Part model, mm, in its own coordinate system. Face numbers are marked on the shaded views. A direction names the side the tool comes from. Coordinates: 2 decimals unless noted, no trailing zeros. Order: outer loops, then holes, each group sorted by start corner. A loop starts at its lowest first (then second) coordinate and runs counter-clockwise, first axis right, second up. Notation, with made-up numbers: M 72,70 L 102,70 A5 ccw 102,76 Z; hole C 31.5,21 d3. An arc over 180 degrees is marked long. Write item = value, one per line. Start each with the question number.
Autodesk Inventor part; units mm, degrees
ref_plane "YZ Plane" through (0, 0, 0) normal (1, 0, 0) x (0, 1, 0)
ref_plane "XZ Plane" through (0, 0, 0) normal (0, 1, 0) x (-1, 0, 0)
ref_plane "XY Plane" through (0, 0, 0) normal (0, 0, 1) x (1, 0, 0)
sketch "Skizze1" plane through (0, 0, 0) normal (0, 1, 0) x (-1, 0, 0)
  line L0 (-10, -5.25) -> (10, -5.25)
  line L1 (10, -5.25) -> (10, 5.25)
  line L2 (10, 5.25) -> (-10, 5.25)
  line L3 (-10, 5.25) -> (-10, -5.25)
  line L4 (-10, -5.25) -> (10, 5.25) construction
  line L5 (10, -5.25) -> (-10, 5.25) construction
  circle A0 centre (4.75, 2.25) radius 1.25
  circle A1 centre (-4.75, 2.25) radius 1.25
  point P0 (0, 0)
  dimension "d0" = 20
  dimension "d1" = 10.5
  dimension "d4" = 2.5
  dimension "d5" = 2.5
  dimension "d6" = 4.75
  dimension "d7" = 3
  dimension "d8" = 3
  dimension "d9" = 4.75
extrude "Extrusion1" add sketch "Skizze1" along normal mid plane 6
sketch "Skizze2" plane through (0, 0, 0) normal (0, 1, 0) x (-1, 0, 0)
  line L0 (10, -5.25) -> (10, 5.25)
  line L1 (10, 5.25) -> (-10, 5.25)
  line L2 (-10, 5.25) -> (-10, -5.25)
  line L3 (-10, -5.25) -> (10, -5.25)
  circle A0 centre (4.75, 2.25) radius 1.25
  circle A1 centre (-4.75, 2.25) radius 1.25
  line L4 (10, 5.25) -> (-10, 5.25)
  line L5 (8.2, 5.25) -> (7.7, 5.25)
  line L6 (7.7, 5.25) -> (7.7, 9.25)
  line L7 (7.7, 9.25) -> (8.2, 9.25)
  line L8 (8.2, 9.25) -> (8.2, 5.25)
  line L9 (0.3746, 5.25) -> (-0.1254, 5.25)
  line L10 (-0.1254, 5.25) -> (-0.1254, 9.25)
  line L11 (-0.1254, 9.25) -> (0.3746, 9.25)
  line L12 (0.3746, 9.25) -> (0.3746, 5.25)
  line L13 (-7.7, 5.25) -> (-8.2, 5.25)
  line L14 (-8.2, 5.25) -> (-8.2, 9.25)
  line L15 (-8.2, 9.25) -> (-7.7, 9.25)
  line L16 (-7.7, 9.25) -> (-7.7, 5.25)
  point P0 (0, 0)
  dimension "d10" = 0.5
  dimension "d11" = 4
  dimension "d12" = 1.8
  dimension "d13" = 1.8
  dimension "d14" = 0.5
  dimension "d15" = 0.5
extrude "Extrusion2" add sketch "Skizze2" along normal mid plane 3.2 contours L1 L6 L7 L8 | L14 L15 L16 L1 | L1 L10 L11 L12
sketch "Skizze3" plane through (0, 0, 0) normal (0, 1, 0) x (-1, 0, 0)
  line L0 (10, -5.25) -> (10, 5.25)
  line L1 (10, 5.25) -> (-10, 5.25)
  line L2 (-10, 5.25) -> (-10, -5.25)
  line L3 (-10, -5.25) -> (10, -5.25)
  circle A0 centre (4.75, 2.25) radius 1.25
  circle A1 centre (-4.75, 2.25) radius 1.25
  line L4 (10, -5.25) -> (-10, -5.25)
  line L5 (-7.1, -5.25) -> (9.9766, -10.265)
  line L6 (9.9766, -10.265) -> (9.1627, -13.0362)
  line L7 (9.1627, -13.0362) -> (10.7453, -13.501)
  line L8 (10.7453, -13.501) -> (11.7, -10.25)
  line L9 (11.7, -10.25) -> (-5.3255, -5.25)
  point P0 (0, 0)
  dimension "d18" = 2.9
  dimension "d19" = 0.5
  dimension "d20" = 1.7
  dimension "d21" = 5
extrude "Extrusion3" add sketch "Skizze3" along normal mid plane 3.4 contours L9 L8 L7 L6 L5 L3
sketch "Skizze4" plane through (0, 0, 0) normal (0, 1, 0) x (-1, 0, 0)
  line L0 (11.7, -10.25) -> (-5.3255, -5.25)
  line L1 (-7.1, -5.25) -> (-5.3255, -5.25)
  line L2 (-7.1, -5.25) -> (9.9766, -10.265)
  line L3 (9.9766, -10.265) -> (9.1627, -13.0362)
  line L4 (9.1627, -13.0362) -> (10.7453, -13.501)
  line L5 (10.7453, -13.501) -> (11.7, -10.25)
  circle A0 centre (10.3631, -11.8755) radius 2.3
  point P0 (0, 0)
  dimension "d24" = 4.6
extrude "Extrusion4" add sketch "Skizze4" along normal mid plane 3 contours L5 L4 L3 L2 A0 L0 | L0 A0 L2 L3 L4 L5
properties part number "00_Endstop_mechanical_vuniversum_microswitch_roll"
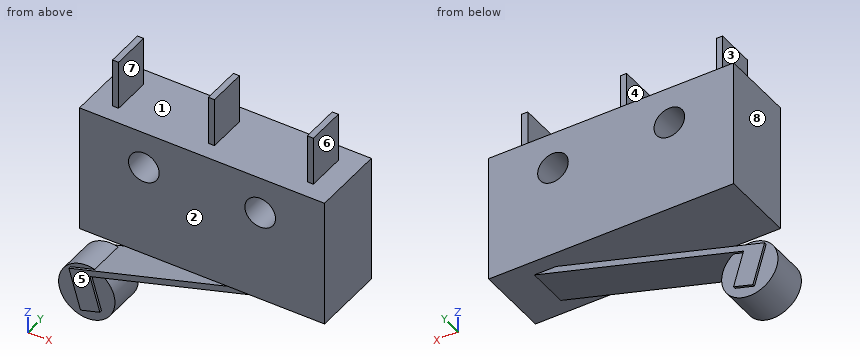
Item 1: Cut at C-C, the plane y = -2.3. Write the cut outline in (x, z).
Item 2: Wall check: line 1 along Z through (x, y) = (4.75, -0.1); line 2 along Z through (x, y) = (-4.75, -0.6); line 3 along X through (y, z) = (2.3, -2.75). Give the ranges that are in metal, low to high. Write a range as [from, to].
Item 3: Flat gauge pins, fed straight in: pin 1 (2.5 mm diameter, centred on x = -10.5, z = -12.5, fed in from +Y); pin 2 (1.6 mm diameter, centred on y = 0.5, z = 6.5, fed in from -X); pin 3 (3 mm diameter, centred on x = 1.5, y = 0, fed in from -Z). Where does each tip first touch, or does it go through?
Item 4: Cut at A-A, the plane z = 7. Write the cut outline in (x, y).
Item 5: 3-axis set-ups, long thin cutter, end or side, ignore diameter. For the marked faces 5, 6, 7 and 8: which of +Z, -Z, +X, -X, +Y, -Y reach the whole face in a straight line?
Item 6: Cut at B-B, the plane x = 4.75. Write the cut outline in (y, z), and give its area (3 significant figures).
Item 7: Cut at D-D, the plane x = -6.5. Write the cut outline in (y, z).
Item 8: Pull direction X, two halves, no side cores. Call the marked faces 1, 2, 3 and 4: pulls with the +X half, pulls with the -X half, needs draft (parallel to the pull), parting line crosses it, or undercut.
Filled sheet:
q1.outline = M -10,-5.25 L 10,-5.25 L 10,5.25 L -10,5.25 Z; hole C -4.75,2.25 d2.5; hole C 4.75,2.25 d2.5
q2.line_1 = [-5.94, -5.42], [-5.25, 1], [3.5, 5.25]
q2.line_2 = [-8.73, -8.21], [-5.25, 1], [3.5, 5.25]
q2.line_3 = [-10, 10]
q3.pin_1 = 1.7
q3.pin_2 = -8.2
q3.pin_3 = -7.34
q4.outline = M -8.2,-1.6 L -7.7,-1.6 L -7.7,1.6 L -8.2,1.6 Z; M -0.37,-1.6 L 0.13,-1.6 L 0.13,1.6 L -0.37,1.6 Z; M 7.7,-1.6 L 8.2,-1.6 L 8.2,1.6 L 7.7,1.6 Z
q5.face_5 = -Z, +X, -X, -Y
q5.face_6 = +Z, +X, +Y, -Y
q5.face_7 = +Z, +Y, -Y
q5.face_8 = +Z, -X, +Y, -Y
q6.outline = M -3,-5.25 L 3,-5.25 L 3,1 L -3,1 Z; M -3,3.5 L 3,3.5 L 3,5.25 L -3,5.25 Z; M -1.7,-5.94 L 1.7,-5.94 L 1.7,-5.42 L -1.7,-5.42 Z
q6.area = 49.8 mm2
q7.outline = M -3,-5.25 L 3,-5.25 L 3,5.25 L -3,5.25 Z; M -1.7,-9.24 L 1.7,-9.24 L 1.7,-8.72 L -1.7,-8.72 Z
q8.face_1 = undercut
q8.face_2 = needs draft
q8.face_3 = pulls with the -X half
q8.face_4 = undercut
